Source: three-view drawing plus pictorial views. Frame: mm from the lowest corner of the part. A direction names the side the tool comes from. Round coordinates to 2 decimals unless told otherwise and drop trailing zeros. Loops run counter-clockwise (first coordinate to the right, second up) from the corner with the lowest first, then second, coordinate; pieces in that order, holes last. Notation, with made-up numbers: M 5.25,-22.75 L 34.25,-22.75 A26 ccw 34.25,9.25 Z; hole C 79,45 d11. An arc over 180 degrees is marked long. Write each question's results on one line, items separated by ' | '.
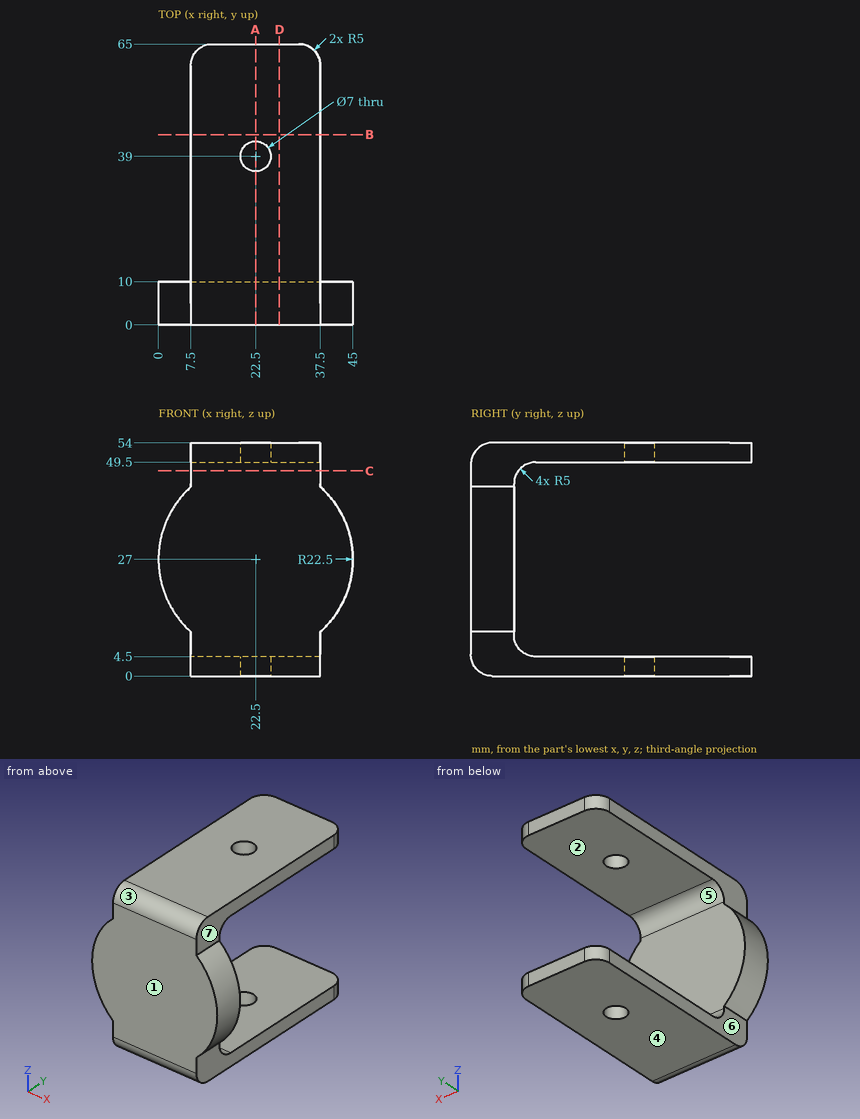
1. Access query for the marked faces 5, 6 and 7. Directions: +Z, -Z, +X, -X, +Y, -Y. A direction counts if a zero-diameter tool reaches every point of the face in a straight line with its end or side. Return the directions, or none.
Answer key:
face 5: +X, -X, +Y | face 6: -Z, -X, +Y, -Y | face 7: +Z, +X, +Y, -Y
2. Section C-C (z = 47.5). Output: boundary loops of the cut face in (x, y).
Answer key:
outline: M 7.5,0 L 37.5,0 L 37.5,11 L 7.5,11 Z
3. Section A-A (x = 22.5). Output: boundary loops of the cut face in (y, z).
Answer key:
outline: M 0,5 A5 ccw 5,0 L 35.5,0 L 35.5,4.5 L 15,4.5 A5 cw 10,9.5 L 10,44.5 A5 cw 15,49.5 L 35.5,49.5 L 35.5,54 L 5,54 A5 ccw 0,49 Z; M 42.5,0 L 65,0 L 65,4.5 L 42.5,4.5 Z; M 42.5,49.5 L 65,49.5 L 65,54 L 42.5,54 Z
4. Ray query, probe 1 along Z at (x, y) = (29, 19); probe 2 along Y at (x, z) = (31.5, 44.5); probe 3 along Y at (x, z) = (22, 52). Return the intervals inside material, ascending.
Answer key:
probe 1: z = 0 to 4.5, 49.5 to 54 | probe 2: y = 0 to 10 | probe 3: y = 1 to 35.54, 42.46 to 65
5. Section B-B (y = 44). Output: boundary loops of the cut face in (x, z).
Answer key:
outline: M 7.5,0 L 37.5,0 L 37.5,4.5 L 7.5,4.5 Z; M 7.5,49.5 L 37.5,49.5 L 37.5,54 L 7.5,54 Z
6. Section D-D (x = 28). Output: boundary loops of the cut face in (y, z), then the cut area to 4 significant figures.
Answer key:
outline: M 0,5 A5 ccw 5,0 L 65,0 L 65,4.5 L 15,4.5 A5 cw 10,9.5 L 10,44.5 A5 cw 15,49.5 L 65,49.5 L 65,54 L 5,54 A5 ccw 0,49 Z | area: 1,035 mm²
7. Pin query (flat end, axial travel): P1, Ø10, axis at x = 26.5, z = 28, coming from the +Y side; P2, Ø11.5, axis at y = 30, z = 50, coming from the +X side; P3, Ø8, axis at y = 22, z = 50, coming from the -X side. Return the tip coordinate at first contact, or that it passes through.
Answer key:
P1: stops at y = 10 | P2: stops at x = 37.5 | P3: stops at x = 7.5
8. Draft query along Z for the marked faces 1, 2, 3 and 4. Return one class per face: pulls with the +Z half, pulls with the -Z half, needs draft (parallel to the pull), parting line crosses it, or undercut.
Answer key:
face 1: needs draft | face 2: undercut | face 3: pulls with the +Z half | face 4: pulls with the -Z half
